Input: part model. Units: mm. Frame: model coordinates. Coordinates: 2 decimals unless noted, no trailing zeros. Loops run counter-clockwise (first coordinate to the right, second up) from the corner with the lowest first, then second, coordinate; pieces in that order, holes last. Notation, with made-up numbers: (-40, 80) -> (-21, 80) arc R9 ccw to (-21, 92) -> close; hole circle Ø7 at (-25.5, -23). An arc over 180 degrees is marked (long way). Put each result on its own line as item: value. Start each with the question number.
1) Pull-direction query (Y, two-part tool) for faces 1 (the cylindrical face through (-55.431, -42.503, -0.178)), 2 (the cylindrical face through (-54.6, -27.6, -0.2)), 3 (the flat face through (-6, 57, 12.7)); classes: pulls with the +Y half, pulls with the -Y half, needs draft (parallel to the pull), parting line crosses it, or undercut.
2) Contact query for flat-ended pins moving along their axis: P1, Ø8, axis at y = -47, z = 2.5, coming from the -X side; P2, Ø12, axis at x = 47.5, z = -4, coming from the +Y side; P3, Ø12, axis at y = -16.5, z = 8, coming from the -X side. Output: stop coordinate, or through.
3) Material intervals for L1, parallel to X at y = 25.5, z = -1.5; L2, parallel to Y at x = 0, z = -6.25; L3, parallel to Y at x = -14, z = -6, sorted ascending.
4) Cut plane A-A (x = 0). Return the cut outline in (y, z), plus the area to 3 significant figures.
5) Cut plane C-C (z = -2). Return the cut outline in (x, y), plus the area to 3 significant figures.
from build123d import *

# Parameters (mm, degrees)
BOSS_EXTRUDE1_DEPTH            = 12.7
BOSS_EXTRUDE1_DEPTH_BACK       = 12.7
SKETCH3_R                      = 69.85
SKETCH3_R_2                    = 57.15
TAP_DRILL_FOR_1_4_20_TAP1_D    = 5.1054
F_5_16_0_3125_DIAMETER_HOLE1_D = 7.9375
CIRPATTERN1_COUNT              = 2


with BuildPart() as part:
    # Sketch3 → Boss-Extrude1 (new, two sides: drawn at the far end of the back side and taken through both)
    with BuildSketch(Plane.XY.offset(-BOSS_EXTRUDE1_DEPTH_BACK)):
        Circle(SKETCH3_R)
        Circle(SKETCH3_R_2, mode=Mode.SUBTRACT)
    extrude(amount=BOSS_EXTRUDE1_DEPTH + BOSS_EXTRUDE1_DEPTH_BACK)

    # Tap Drill for 1/4-20 Tap1 (through all)
    with Locations(Plane.XY.offset(12.7)):
        with Locations((-57.15, -27.679008291), (-62.366515468, -11.944360527)):
            tap_drill_for_1_4_20_tap1 = Hole(TAP_DRILL_FOR_1_4_20_TAP1_D / 2)

    # 5/16 (0.3125) Diameter Hole1 (through all)
    with Locations(Plane.XY.offset(12.7)):
        with Locations((-12.413435939, -62.274847316)):
            f_5_16_0_3125_diameter_hole1 = Hole(F_5_16_0_3125_DIAMETER_HOLE1_D / 2)

    # CirPattern1: Tap Drill for 1/4-20 Tap1, 5/16 (0.3125) Diameter Hole1 ×2 about axis
    cirpattern1_axis = Axis((0, 0, 0), (0, 0, 1))
    add([tap_drill_for_1_4_20_tap1.rotate(cirpattern1_axis, i * 360 / CIRPATTERN1_COUNT) for i in range(1, CIRPATTERN1_COUNT)], mode=Mode.SUBTRACT)
    add([f_5_16_0_3125_diameter_hole1.rotate(cirpattern1_axis, i * 360 / CIRPATTERN1_COUNT) for i in range(1, CIRPATTERN1_COUNT)], mode=Mode.SUBTRACT)


solid = part.part
Results found:
1. face 1: parting line crosses it
1. face 2: undercut
1. face 3: needs draft
2. P1: stops at x = -55.05
2. P2: stops at y = 56.19
2. P3: stops at x = -69.06
3. L1: x = -65.03 to -51.15, 51.15 to 55.82, 58.48 to 65.03
3. L2: y = -69.85 to -57.15, 57.15 to 69.85
3. L3: y = -68.43 to -65.91, -58.64 to -55.41, 55.41 to 68.43
4. outline: (-69.85, -12.7) -> (-57.15, -12.7) -> (-57.15, 12.7) -> (-69.85, 12.7) -> close; (57.15, -12.7) -> (69.85, -12.7) -> (69.85, 12.7) -> (57.15, 12.7) -> close
4. area: 645 mm2
5. outline: circle Ø139.7 at (0, 0); hole circle Ø5.11 at (-62.37, -11.94); hole circle Ø5.11 at (-57.15, -27.68); hole circle Ø114.3 at (0, 0); hole circle Ø7.94 at (-12.41, -62.27); hole circle Ø7.94 at (12.41, 62.27); hole circle Ø5.11 at (57.15, 27.68); hole circle Ø5.11 at (62.37, 11.94)
5. area: 4,890 mm2
